```python
from build123d import *

# Parameters (mm, degrees)
F1_DEPTH       = 250
F2_W           = 38
F2_H           = 13
F3_DEPTH       = 250
F4_T1_DEPTH    = 509.3674969976
F5_R           = 9
F6_R           = 1
F8_DEPTH       = 500.001
F10_DEPTH      = 24.4523840141
F10_DEPTH_BACK = 527
F12_DEPTH      = 527
F12_DEPTH_BACK = 24.4523841141
F13_F1_R       = 4.9999
F13_F2_R       = 4.9999
F13_F3_R       = 5
F13_F4_R       = 5
F13_F5_R       = 5
F13_F6_R       = 5
F15_DEPTH      = 15
F16_R          = 27.4590604355
F17_DEPTH      = 100
F19_D          = 40
F21_D          = 8
F21_DEPTH      = 50
F21_TIP        = 2.4034424761


# Not quite as in the source:
# - a fillet or chamfer that OpenCascade refuses, or shapes differently, is made with other operations: its cross-section is extruded or revolved along the edge and cut away or added
# - a fillet or chamfer is up to 0.001 mm smaller than in the source, because OpenCascade refuses the exact size
# - an extrude ends at something that could not be found from the text; its depth is read off the source's solid


with BuildPart() as f1:
    # F0 (on Front) → F1 (new body, symmetric)
    with BuildSketch(Plane.XZ):
        with BuildLine():
            Line((22.5, 23.1513840141), (0, 23.1513840141))
            Line((0, 23.1513840141), (-22.5, 23.1513840141))
            Line((-22.5, 23.1513840141), (-22.5, 24.4513840141))
            Line((-22.5, 24.4513840141), (-45.5824640741, 24.4513840141))
            Line((-45.5824640741, 24.4513840141), (-57.5, 14.4513840141))
            Line((-57.5, 14.4513840141), (-57.5, 10.4513840141))
            Line((-57.5, 10.4513840141), (-40.1794919243, 0.4513840141))
            ThreePointArc((-40.1794919243, 0.4513840141), (0, 4.5289288725), (40.1794919243, 0.4513840141))
            Line((40.1794919243, 0.4513840141), (57.5, 10.4513840141))
            Line((57.5, 10.4513840141), (57.5, 14.4513840141))
            Line((57.5, 14.4513840141), (45.5824640741, 24.4513840141))
            Line((45.5824640741, 24.4513840141), (22.5, 24.4513840141))
            Line((22.5, 24.4513840141), (22.5, 23.1513840141))
        make_face()
    extrude(amount=F1_DEPTH, both=True)

    # F2 (on Front) → F3 (cut, symmetric)
    with BuildSketch(Plane.XZ):
        with Locations((0, 14.6513840141)):
            Rectangle(F2_W, F2_H)
    extrude(amount=F3_DEPTH, both=True, mode=Mode.SUBTRACT)

    # F4: fillet of radius 2 on 2 edges, made by hand

    # F4_s2 → F4_t1 (cut)
    with BuildSketch(Plane.XZ.offset(-254.6837484988)):
        with BuildLine():
            ThreePointArc((-24.3734993995, 24.4513840141), (-23.2333239744, 24.0945516866), (-22.5, 23.1513840141))
            Line((-22.5, 23.1513840141), (-22.5, 24.4513840141))
            Line((-22.5, 24.4513840141), (-24.3734993995, 24.4513840141))
        make_face()
        with BuildLine():
            ThreePointArc((24.3734993995, 24.4513840141), (23.2333239744, 24.0945516866), (22.5, 23.1513840141))
            Line((22.5, 23.1513840141), (22.5, 24.4513840141))
            Line((22.5, 24.4513840141), (24.3734993995, 24.4513840141))
        make_face()
    extrude(amount=F4_T1_DEPTH, mode=Mode.SUBTRACT)

    # F5
    f5_edges = [f1.edges().sort_by_distance(p)[0] for p in [
        (-45.582464, 0, 24.451384),
        (-40.179492, 0, 0.451384),
        (40.179492, 0, 0.451384),
        (45.582464, 0, 24.451384),
    ]]
    fillet(f5_edges, radius=F5_R)

    # F6
    f6_edges = [f1.edges().sort_by_distance(p)[0] for p in [
        (57.5, 0, 14.451384),
        (57.5, 0, 10.451384),
        (-57.5, 0, 10.451384),
        (-57.5, 0, 14.451384),
    ]]
    fillet(f6_edges, radius=F6_R)

    # F7 (on face) → F8 (cut, through all)
    with BuildSketch(Plane.XZ.offset(250)):
        with BuildLine():
            ThreePointArc((-42.1022690923, 3.8709010064), (-39.7790673433, 3.0327059534), (-37.3093701274, 3.0535140017))
            ThreePointArc((-37.3093701274, 3.0535140017), (-29.1789785809, 4.4103617496), (-21, 5.4343792715))
            Line((-21, 5.4343792715), (-21, 21.1513840141))
            Line((-21, 21.1513840141), (-22.5, 21.1513840141))
            ThreePointArc((-22.5, 21.1513840141), (-23.2333239744, 22.0945516866), (-24.3734993995, 22.4513840141))
            Line((-24.3734993995, 22.4513840141), (-42.3067319657, 22.4513840141))
            ThreePointArc((-42.3067319657, 22.4513840141), (-44.7008729689, 22.0292323596), (-46.8062452335, 20.813695116))
            Line((-46.8062452335, 20.813695116), (-55.7563117574, 13.3036975967))
            ThreePointArc((-55.7563117574, 13.3036975967), (-56.1097188459, 12.4504974108), (-55.6135241478, 11.6716277498))
            Line((-55.6135241478, 11.6716277498), (-42.1022690923, 3.8709010064))
        make_face()
        with BuildLine():
            Line((21, 21.1513840141), (21, 5.4343792715))
            ThreePointArc((21, 5.4343792715), (29.1789785809, 4.4103617496), (37.3093701274, 3.0535140017))
            ThreePointArc((37.3093701274, 3.0535140017), (39.7790673433, 3.0327059534), (42.1022690923, 3.8709010064))
            Line((42.1022690923, 3.8709010064), (55.6135241478, 11.6716277498))
            ThreePointArc((55.6135241478, 11.6716277498), (56.1097188459, 12.4504974108), (55.7563117574, 13.3036975967))
            Line((55.7563117574, 13.3036975967), (46.8062452335, 20.813695116))
            ThreePointArc((46.8062452335, 20.813695116), (44.7008729689, 22.0292323596), (42.3067319657, 22.4513840141))
            Line((42.3067319657, 22.4513840141), (24.3734993995, 22.4513840141))
            ThreePointArc((24.3734993995, 22.4513840141), (23.2333239744, 22.0945516866), (22.5, 21.1513840141))
            Line((22.5, 21.1513840141), (21, 21.1513840141))
        make_face()
    extrude(amount=-F8_DEPTH, mode=Mode.SUBTRACT)

    # F9 (on Top) → F10 (cut, two sides)
    with BuildSketch(Plane.XY) as f10_sk:
        with BuildLine():
            ThreePointArc((-57.5, 200), (0, 257.5), (57.5, 200))
            Line((57.5, 200), (57.5, 280))
            Line((57.5, 280), (-57.5, 280))
            Line((-57.5, 280), (-57.5, 200))
        make_face()
    extrude(amount=F10_DEPTH, mode=Mode.SUBTRACT)
    extrude(f10_sk.sketch, amount=-F10_DEPTH_BACK, mode=Mode.SUBTRACT)

    # F11 (on Top) → F12 (cut, two sides)
    with BuildSketch(Plane.XY) as f12_sk:
        Polygon((-43.2975540478, -250), (-68, -216), (-68, -346), (68, -346), (68, -216), (43.2975540478, -250), (16, -250), (16, -140), (-16, -140), (-16, -250), align=None)
    extrude(amount=-F12_DEPTH, mode=Mode.SUBTRACT)
    extrude(f12_sk.sketch, amount=F12_DEPTH_BACK, mode=Mode.SUBTRACT)

    # F13: fillet of radius 5 on 8 edges, made by hand

    # F13_f1 (radius 5 in the source; OpenCascade refuses exactly that, so slightly less here)
    f13_f1_edges = [f1.edges().sort_by_distance(p)[0] for p in [
        (-16, -250, 22.1513840141),
    ]]
    fillet(f13_f1_edges, radius=F13_F1_R)

    # F13_f2 (radius 5 in the source; OpenCascade refuses exactly that, so slightly less here)
    f13_f2_edges = [f1.edges().sort_by_distance(p)[0] for p in [
        (16, -250, 6.0196427984),
    ]]
    fillet(f13_f2_edges, radius=F13_F2_R)

    # F13_f3
    f13_f3_edges = [f1.edges().sort_by_distance(p)[0] for p in [
        (16, -140, 22.1513840141),
    ]]
    fillet(f13_f3_edges, radius=F13_F3_R)

    # F13_f4
    f13_f4_edges = [f1.edges().sort_by_distance(p)[0] for p in [
        (-16, -140, 22.1513840141),
    ]]
    fillet(f13_f4_edges, radius=F13_F4_R)

    # F13_f5
    f13_f5_edges = [f1.edges().sort_by_distance(p)[0] for p in [
        (-16, -140, 6.0196427984),
    ]]
    fillet(f13_f5_edges, radius=F13_F5_R)

    # F13_f6
    f13_f6_edges = [f1.edges().sort_by_distance(p)[0] for p in [
        (16, -140, 6.0196427984),
    ]]
    fillet(f13_f6_edges, radius=F13_F6_R)

    # F14 (on Right) → F15 (join, symmetric)
    with BuildSketch(Plane.YZ):
        with BuildLine():
            ThreePointArc((297.3819995028, 183.1513840141), (245.9666940414, 97.8136618671), (180, 23.1513840141))
            Line((180, 23.1513840141), (250, 23.1513840141))
            ThreePointArc((250, 23.1513840141), (267.6550746197, 69.6272787008), (311.7145367693, 92.6593051387))
            Line((311.7145367693, 92.6593051387), (313.0254460068, 84.3825499546))
            Line((313.0254460068, 84.3825499546), (358.4591096742, 91.5785353465))
            Line((358.4591096742, 91.5785353465), (342.8156631702, 190.347369406))
            Line((342.8156631702, 190.347369406), (297.3819995028, 183.1513840141))
        make_face()
    extrude(amount=F15_DEPTH, both=True)

    # F16 (on face) → F17 (join, through all)
    with BuildSketch(Plane(origin=(0, -21.0209895784, 132.7213047908), x_dir=(1, 0, 0), z_dir=(0, -0.156434465, 0.9876883406))):
        with Locations((0, 345.3719223914)):
            Circle(F16_R)
    extrude(amount=-F17_DEPTH)

    # F19 (through all)
    with Locations(Plane(origin=(0, -21.0209895784, 132.7213047908), x_dir=(1, 0, 0), z_dir=(0, -0.156434465, 0.9876883406))):
        with Locations((0, 345.3719223914)):
            Hole(F19_D / 2)

    # F21 (one way)
    with BuildSketch(Plane.YZ.offset(21)):
        with Locations((-236, 15.4343792715)):
            Circle(F21_D / 2)
    extrude(amount=-F21_DEPTH, mode=Mode.SUBTRACT)
    with Locations(Plane.YZ.offset(21)):
        with Locations((-236, 15.4343792715)):
            with Locations((0, 0, -(F21_DEPTH + F21_TIP / 2))):  # 118° drill point
                Cone(0, F21_D / 2, F21_TIP, mode=Mode.SUBTRACT)


solid = f1.part
```
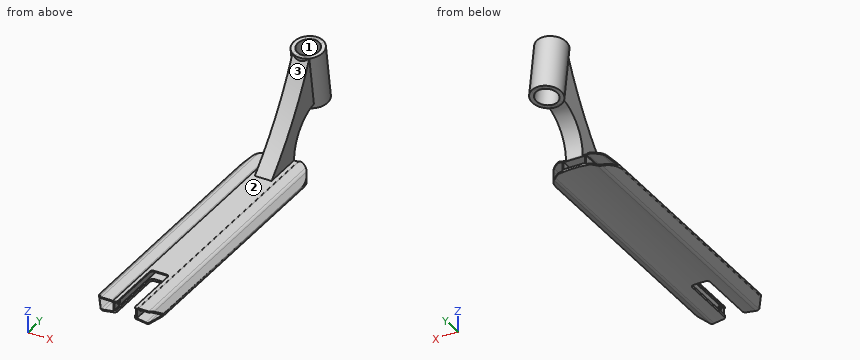
Geometry: final body of the model. Coordinates: model frame, mm. Face numbers are marked on the shaded views. Round coordinates to 2 decimals unless told otherwise and drop trailing zeros. Loops run counter-clockwise (first coordinate to the right, second up) from the corner with the lowest first, then second, coordinate; pieces in that order, holes last. Notation, with made-up numbers: (20.25, 65) -> (58.25, 65) arc R27 ccw to (58.25, 94) -> close; hole circle Ø7 at (83, 60.5). An arc over 180 degrees is marked (long way). Write each question's results on one line, items separated by ' | '.
Item 1: Pull-direction query (Y, two-part tool) for the marked faces 1, 2 and 3; classes: pulls with the +Y half, pulls with the -Y half, needs draft (parallel to the pull), parting line crosses it, or undercut.
Answers below:
face 1: undercut | face 2: needs draft | face 3: pulls with the -Y half
Item 2: Cut plane A-A on y = 62. State how many separate pieces and enclosed holes the cut face has, and give its area (3 significant figures).
Answers below:
separate pieces: 1 | enclosed holes: 3 | area: 621 mm²
Item 3: Cut plane B-B on z = 60. Return the cut outline in (x, y), and give its area (3 significant figures).
Answers below:
outline: (-15, 215.57) -> (15, 215.57) -> (15, 260.48) -> (-15, 260.48) -> close | area: 1,350 mm²
Item 4: Line query: probe 1 along Z at (x, y) = (10.5, -81); probe 2 along Z at (x, y) = (-19.7, -236); probe 3 along X at (y, z) = (-191, 21). Output: solid intervals per line, ascending. Write a range as [from, to].
Answers below:
probe 1: z = [4.25, 8.15], [21.15, 23.15] | probe 2: z = [3.56, 11.43], [19.43, 23.15] | probe 3: x = [-49.7, -46.57], [-21, -19], [19, 21], [46.57, 49.7]
Item 5: Pin query (flat end, axial travel): pin 1 Ø9 at (x, y) = (-31, 39) entering from -Z; pin 2 Ø6.5 at (y, z) = (-85.5, 17.5) entering from +X; pin 3 Ø1 at (y, z) = (-175, 22) entering from +X. Return the tip coordinate at first contact, or that it passes through.
Answers below:
pin 1: stops at z = 1.35 | pin 2: stops at x = 57.46 | pin 3: stops at x = 49.1
